```python
from build123d import *

# Parameters (mm, degrees)
BOSS_EXTRUDE1_DEPTH = 28
SKETCH3_W           = 19
SKETCH3_H           = 28
CUT_EXTRUDE1_DEPTH  = 30.5
SKETCH4_W           = 3
SKETCH4_H           = 30
CUT_EXTRUDE2_DEPTH  = 2
CUT_EXTRUDE3_DEPTH  = 36
SKETCH6_W           = 7
SKETCH6_H           = 23
CUT_EXTRUDE4_DEPTH  = 2
SKETCH11_W          = 29.75
SKETCH11_H          = 3
SKETCH11_W_2        = 23
SKETCH11_H_2        = 7
CUT_EXTRUDE6_DEPTH  = 2
CUT_EXTRUDE7_DEPTH  = 34


with BuildPart() as part:
    # Sketch1 → Boss-Extrude1 (new body)
    with BuildSketch(Plane.XY):
        Polygon((0, 0), (35, 0), (35, 35), (28, 35), (28, 32), (3, 7), (0, 7), align=None)
    extrude(amount=BOSS_EXTRUDE1_DEPTH)

    # Sketch3 → Cut-Extrude1 (cut)
    with BuildSketch(Plane.ZY):
        with Locations((14, 21)):
            Rectangle(SKETCH3_W, SKETCH3_H)
    extrude(amount=-CUT_EXTRUDE1_DEPTH, mode=Mode.SUBTRACT)

    # Sketch4 → Cut-Extrude2 (cut)
    with BuildSketch(Plane(origin=(35, 0, 0), x_dir=(0, 0, -1), z_dir=(1, 0, 0))):
        with Locations((-24, 17.75)):
            Rectangle(SKETCH4_W, SKETCH4_H)
        with Locations((-4, 17.75)):
            Rectangle(SKETCH4_W, SKETCH4_H)
    extrude(amount=-CUT_EXTRUDE2_DEPTH, mode=Mode.SUBTRACT)

    # Sketch5 → Cut-Extrude3 (cut, through all)
    with BuildSketch(Plane(origin=(35, 0, 0), x_dir=(0, 0, -1), z_dir=(1, 0, 0))):
        with BuildLine():
            Line((-10.5, 23.25), (-10.5, 11.75))
            ThreePointArc((-10.5, 11.75), (-14, 8.25), (-17.5, 11.75))
            Line((-17.5, 11.75), (-17.5, 23.25))
            ThreePointArc((-17.5, 23.25), (-14, 26.75), (-10.5, 23.25))
        make_face()
    extrude(amount=-CUT_EXTRUDE3_DEPTH, mode=Mode.SUBTRACT)

    # Sketch6 → Cut-Extrude4 (cut)
    with BuildSketch(Plane(origin=(35, 0, 0), x_dir=(0, 0, -1), z_dir=(1, 0, 0))):
        with Locations((-14, 17.5)):
            Rectangle(SKETCH6_W, SKETCH6_H)
    extrude(amount=-CUT_EXTRUDE4_DEPTH, mode=Mode.SUBTRACT)

    # Sketch11 → Cut-Extrude6 (cut)
    with BuildSketch(Plane.XZ):
        with Locations((17.375, 24)):
            Rectangle(SKETCH11_W, SKETCH11_H)
        with Locations((17.375, 4)):
            Rectangle(SKETCH11_W, SKETCH11_H)
        with Locations((17.5, 14)):
            Rectangle(SKETCH11_W_2, SKETCH11_H_2)
    extrude(amount=-CUT_EXTRUDE6_DEPTH, mode=Mode.SUBTRACT)

    # Sketch12 → Cut-Extrude7 (cut, through all)
    with BuildSketch(Plane.XZ.offset(-2)):
        with BuildLine():
            Line((11.75, 17.5), (23.25, 17.5))
            ThreePointArc((23.25, 17.5), (26.75, 14), (23.25, 10.5))
            Line((23.25, 10.5), (11.75, 10.5))
            ThreePointArc((11.75, 10.5), (8.25, 14), (11.75, 17.5))
        make_face()
    extrude(amount=-CUT_EXTRUDE7_DEPTH, mode=Mode.SUBTRACT)


solid = part.part
```
Geometry: final body of the model. Coordinates: model frame, mm. A direction names the side the tool comes from. Give positions to 0.01 mm unless a question says otherwise; leave off trailing zeros. Loops run counter-clockwise (first coordinate to the right, second up) from the corner with the lowest first, then second, coordinate; pieces in that order, holes last. Notation, with made-up numbers: (67, -2.75) - (120, -2.75) arc R13 cw to (120, 8.25) - close; hole circle Ø6 at (74, 85). An arc over 180 degrees is marked (long way). Answer as CSV lines item,"result". Start each with the question number.
(1) Reachability of faces 5 (the face through (34, 32.75, 4)), 6 (the face through (28, 34, 2)), 7 (the face through (31.77, 8.25, 13.92)), 8 (the face through (6, 1, 14)) from +Z, -Z, +X, -X, +Y, -Y: full face, straight path, thin tool, end or side. Return the list, or none.
(2) Section query C-C (z = 14). Output: boundary loops of the cut face in (x, y).
(3) Section query A-A (y = 20.5). Output: boundary loops of the cut face in (x, z).
(4) Pin query (flat end, axial travel): P1, Ø1.7, axis at y = 27.5, z = 13.5, coming from the +X side; P2, Ø0.9, axis at x = 15.5, z = 4.5, coming from the -Y side. Return the tip coordinate at first contact, or that it passes through.
(5) Section query D-D (x = 27.5). Output: boundary loops of the cut face in (y, z), and give its area (4 significant figures).
(6) Ray query, line 1 along Z through (x, y) = (20.5, 14.5); line 2 along X through (y, z) = (18.5, 9); line 3 along X through (y, z) = (9.5, 25.75). Return the intervals inside material, ascending. Write a range as [from, to].
(7) Mould query, pull axis Z, two halves, no side actions, for faces 1 (the face through (34, 2.75, 24)), 2 (the face through (21, 14, 28)), 3 (the face through (17, 0, 20)), 4 (the face through (30.5, 21, 18)). Classes: +Z half, -Z half, draft (parallel to the pull), parting line (faces both ways), or undercut.
(8) Section query B-B (x = 17). Output: boundary loops of the cut face in (y, z), and give its area (3 significant figures).
Worked answers:
1,face 5,"+X"
1,face 6,"+Z, -Z, -X, +Y"
1,face 7,"+X, -X"
1,face 8,"-Y"
2,outline,"(0, 0) - (6, 0) - (6, 2) - (8.25, 2) - (8.25, 7) - (0, 7) - close; (26.75, 2) - (29, 2) - (29, 0) - (35, 0) - (35, 6) - (33, 6) - (33, 8.25) - (30.5, 8.25) - (30.5, 7) - (26.75, 7) - close; (30.5, 26.75) - (33, 26.75) - (33, 29) - (35, 29) - (35, 35) - (30.5, 35) - close"
3,outline,"(16.5, 0) - (35, 0) - (35, 2.5) - (33, 2.5) - (33, 5.5) - (35, 5.5) - (35, 10.5) - (30.5, 10.5) - (30.5, 4.5) - (16.5, 4.5) - close; (16.5, 23.5) - (30.5, 23.5) - (30.5, 17.5) - (35, 17.5) - (35, 22.5) - (33, 22.5) - (33, 25.5) - (35, 25.5) - (35, 28) - (16.5, 28) - close"
4,P1,"stops at x = 33"
4,P2,"stops at y = 2"
5,outline,"(0, 0) - (31.5, 0) - (31.5, 4.5) - (7, 4.5) - (7, 23.5) - (31.5, 23.5) - (31.5, 28) - (0, 28) - (0, 25.5) - (2, 25.5) - (2, 22.5) - (0, 22.5) - (0, 17.5) - (2, 17.5) - (2, 10.5) - (0, 10.5) - (0, 5.5) - (2, 5.5) - (2, 2.5) - (0, 2.5) - close"
5,area,"390.5 mm^2"
6,line 1,"z = [0, 4.5], [23.5, 28]"
6,line 2,"x = [30.5, 35]"
6,line 3,"x = [5.5, 35]"
7,face 1,"undercut"
7,face 2,"+Z half"
7,face 3,"draft"
7,face 4,"undercut"
8,outline,"(0, 0) - (21, 0) - (21, 4.5) - (7, 4.5) - (7, 10.5) - (0, 10.5) - (0, 5.5) - (2, 5.5) - (2, 2.5) - (0, 2.5) - close; (0, 17.5) - (7, 17.5) - (7, 23.5) - (21, 23.5) - (21, 28) - (0, 28) - (0, 25.5) - (2, 25.5) - (2, 22.5) - (0, 22.5) - close"
8,area,"261 mm^2"
